Source: CAD feature listing. Evaluate the final solid. Frame: model axes, mm. Face numbers are marked on the shaded views. A direction names the side the tool comes from. Give positions to 0.01 mm unless a question says otherwise; leave off trailing zeros. Write each loop counter-clockwise with the first axis right and the second up, starting at its lowest first coordinate (ties: lowest second). Pieces come first, ordered by that corner, then holes.
```python
from build123d import *

# Parameters (mm, degrees)
EXTRUDE_1_DEPTH     = 10
SKETCH_2_R          = 1.6
CUT_EXTRUDE_1_DEPTH = 84.066238629
SKETCH_3_R          = 1.6
CUT_EXTRUDE_2_DEPTH = 4


with BuildPart() as part:
    # 草图1 → 凸台-拉伸1 (new body)
    with BuildSketch(Plane.XY):
        Polygon((0, 0), (20, 0), (20, 20), (80, 20), (80, 11), (30, -6), (0, -6), align=None)
        Polygon((24, 16), (24, 1), (38.162121481, 1), (76, 13.864878696), (76, 16), align=None, mode=Mode.SUBTRACT)
    extrude(amount=EXTRUDE_1_DEPTH)

    # 草图2 → 切除-拉伸1 (cut, through all)
    with BuildSketch(Plane(origin=(0, 0, 0), x_dir=(1, 0, 0), z_dir=(0, 1, 0))):
        with Locations(Location((10, -5, 0), (0, 0, 270))):
            Circle(SKETCH_2_R)
    extrude(amount=-CUT_EXTRUDE_1_DEPTH, mode=Mode.SUBTRACT)

    # 草图3 → 切除-拉伸2 (cut)
    with BuildSketch(Plane(origin=(0, 20, 0), x_dir=(1, 0, 0), z_dir=(0, 1, 0))):
        with Locations(Location((65, -5, 0), (0, 0, 180))):
            Circle(SKETCH_3_R)
        with Locations(Location((35, -5, 0), (0, 0, 180))):
            Circle(SKETCH_3_R)
    extrude(amount=-CUT_EXTRUDE_2_DEPTH, mode=Mode.SUBTRACT)


solid = part.part
```
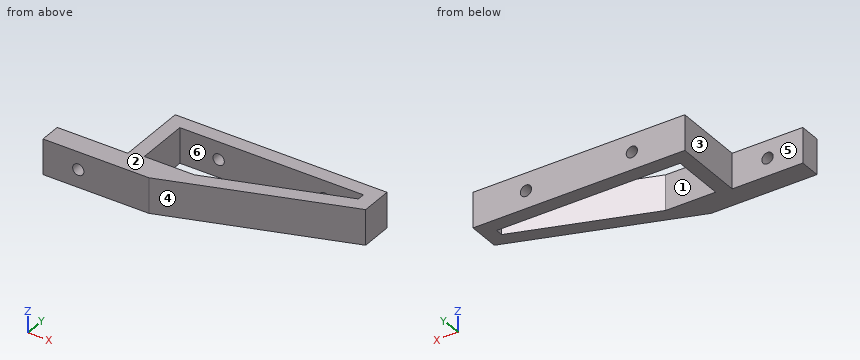
1. Cut plane A-A, the plane x = 35. Return the cut outline in (y, z).
2. Access query for the marked faces 1, 2 and 3. Directions: +Z, -Z, +X, -X, +Y, -Y. A direction counts if a zero-diameter tool reaches every point of the face in a straight line with its end or side. Return the directions, or none.
3. Cut plane C-C, the plane x = 10. Return the cut outline in (y, z).
4. Line query: L1, parallel to X at y = 15, z = 1; L2, parallel to Z at x = 65, y = 18; L3, parallel to Y at x = 13, z = 5.75. Output: solid intervals per line, ascending.
5. Mould query, pull axis Y, two halves, no side actions, for the marked faces 4, 5 and 6. Classes: +Y half, -Y half, draft (parallel to the pull), parting line (faces both ways), or undercut.
6. Contact query for flat-ended pins moving along their axis: P1, Ø3, axis at x = 17, z = 2.5, coming from the +Y side; P2, Ø5, axis at y = 14, z = 7.5, coming from the -X side; P3, Ø8, axis at x = 44.5, y = 3, coming from the -Z side; P4, Ø4, axis at x = 35, z = 5, coming from the -Y side. Output: stop coordinate, or through.
7. Cut plane B-B, the plane z = 5. Return the cut outline in (x, y).
8. Cut plane D-D, the plane z = 0.75. Return the cut outline in (x, y).
Response values:
1. outline: (-4.3, 0) - (1, 0) - (1, 10) - (-4.3, 10) - close; (16, 0) - (20, 0) - (20, 3.4) - (16, 3.4) - close; (16, 6.6) - (20, 6.6) - (20, 10) - (16, 10) - close
2. face 1: +Z, -Z
2. face 2: +Z, +X, -X, +Y, -Y
2. face 3: +Z, -Z, -X, +Y
3. outline: (-6, 0) - (0, 0) - (0, 3.4) - (-6, 3.4) - close; (-6, 6.6) - (0, 6.6) - (0, 10) - (-6, 10) - close
4. L1: x = 20 to 24, 76 to 80
4. L2: z = 0 to 3.4, 6.6 to 10
4. L3: y = -6 to 0
5. face 4: -Y half
5. face 5: +Y half
5. face 6: undercut
6. P1: stops at y = 0
6. P2: stops at x = 20
6. P3: stops at z = 0
6. P4: stops at y = -4.98
7. outline: (0, -6) - (8.4, -6) - (8.4, 0) - (0, 0) - close; (11.6, -6) - (30, -6) - (80, 11) - (80, 20) - (66.6, 20) - (66.6, 16) - (76, 16) - (76, 13.86) - (38.16, 1) - (24, 1) - (24, 16) - (33.4, 16) - (33.4, 20) - (20, 20) - (20, 0) - (11.6, 0) - close; (36.6, 16) - (63.4, 16) - (63.4, 20) - (36.6, 20) - close
8. outline: (0, -6) - (30, -6) - (80, 11) - (80, 20) - (20, 20) - (20, 0) - (0, 0) - close; hole (24, 1) - (38.16, 1) - (76, 13.86) - (76, 16) - (24, 16) - close
